from build123d import *

# Parameters (mm, degrees)
SKETCH1_R                = 7.5
SKETCH1_R_2              = 4
BOSS_EXTRUDE1_DEPTH      = 3
SKETCH2_R                = 8.5
SKETCH2_R_2              = 5.5
BOSS_EXTRUDE2_DEPTH      = 12
CUT_EXTRUDE1_DEPTH       = 17.985287751
CUT_EXTRUDE1_DEPTH_BACK  = 17.985287751
SKETCH4_R                = 1.5
BOSS_EXTRUDE4_DEPTH      = 6
BOSS_EXTRUDE4_DEPTH_BACK = 3
SKETCH5_R                = 8
SKETCH5_R_2              = 7


with BuildPart() as part:
    # Sketch1 → Boss-Extrude1 (new body)
    with BuildSketch(Plane.XY):
        Circle(SKETCH1_R)
        Circle(SKETCH1_R_2, mode=Mode.SUBTRACT)
    extrude(amount=BOSS_EXTRUDE1_DEPTH)

    # Sketch2 → Boss-Extrude2 (add)
    with BuildSketch(Plane.XY):
        Circle(SKETCH2_R)
        Circle(SKETCH2_R_2, mode=Mode.SUBTRACT)
    extrude(amount=-BOSS_EXTRUDE2_DEPTH)

    # Sketch4 → Cut-Extrude1 (cut, two sides: drawn at the far end of the back side and taken through both)
    with BuildSketch(Plane(origin=(0, 0, 0), x_dir=(0, 0, -1), z_dir=(1, 0, 0)).offset(-CUT_EXTRUDE1_DEPTH_BACK)):
        with Locations((7.5, 0)):
            Circle(SKETCH4_R)
    extrude(amount=CUT_EXTRUDE1_DEPTH + CUT_EXTRUDE1_DEPTH_BACK, mode=Mode.SUBTRACT)

    # Sketch5 → Boss-Extrude4 (add, two sides: drawn at the far end of the back side and taken through both)
    with BuildSketch(Plane.XY.offset(3).offset(-BOSS_EXTRUDE4_DEPTH_BACK)):
        Circle(SKETCH5_R)
        Circle(SKETCH5_R_2, mode=Mode.SUBTRACT)
    extrude(amount=BOSS_EXTRUDE4_DEPTH + BOSS_EXTRUDE4_DEPTH_BACK)


solid = part.part
Model file for the job. Use its own axes, mm. A direction names the side the tool comes from. Give positions to 0.01 mm unless a question says otherwise; leave off trailing zeros. Loops run counter-clockwise (first coordinate to the right, second up) from the corner with the lowest first, then second, coordinate; pieces in that order, holes last.
1) Saw through at B-B (x = 0). Write the cut outline in (y, z), plus the area to 3 significant figures.
2) Pull direction X, two halves, no side cores. Call faces 1 (the cylindrical face through (-1.73, -7.81, 4.44)), 2 (the cylindrical face through (-0.867, -3.905, 1.479)), 3 (the cylindrical face through (-6.918, -0.575, -8.886)): +X half, -X half, draft (parallel to the pull), parting line (faces both ways), or undercut.
3) Wall check: line 1 (Z direction, x = 7.4, y = 0); line 2 (X direction, y = 0, z = -4). Give the ranges that are in metal, low to high.
4) Saw through at D-D (z = -2.5). Write the cut outline in (x, y), plus the area to 3 significant figures.
5) Saw through at A-A (y = 0). Write the cut outline in (x, z).
6) Flat gauge pins, fed straight in: pin 1 Ø2 at (x, z) = (5, -5.5) entering from +Y; pin 2 Ø6.5 at (x, y) = (0, 0) entering from -Z; pin 3 Ø1 at (x, z) = (4, -2) entering from -Y; pin 4 Ø3.5 at (x, y) = (1, -2.5) entering from -Z. Where does each tip first touch, or does it go through?
7) Tool access for faces 4 (the flat face through (4, -6, 9)), 5 (the flat face through (-4, -2, 0)), 6 (the flat face through (3, -3, 3)): list every direction of +Z, -Z, +X, -X, +Y, -Y with a clear straight run to the whole face (end or side of a thin tool).
8) Saw through at C-C (z = -6.75). Write the cut outline in (x, y).
Answer block:
1. outline: (-8.5, -12) - (-5.5, -12) - (-5.5, 0) - (-4, 0) - (-4, 3) - (-7, 3) - (-7, 9) - (-8, 9) - (-8, 0) - (-8.5, 0) - close; (4, 0) - (5.5, 0) - (5.5, -12) - (8.5, -12) - (8.5, 0) - (8, 0) - (8, 9) - (7, 9) - (7, 3) - (4, 3) - close
1. area: 108 mm2
2. face 1: parting line
2. face 2: undercut
2. face 3: draft
3. line 1: z = -12 to -9, -6 to 9
3. line 2: x = -8.5 to -5.5, 5.5 to 8.5
4. outline: circle Ø17 at (0, 0); hole circle Ø11 at (0, 0)
4. area: 132 mm2
5. outline: (-8.5, -12) - (-5.5, -12) - (-5.5, -9) - (-8.5, -9) - close; (-8.5, -6) - (-5.5, -6) - (-5.5, 0) - (-4, 0) - (-4, 3) - (-7, 3) - (-7, 9) - (-8, 9) - (-8, 0) - (-8.5, 0) - close; (4, 0) - (5.5, 0) - (5.5, -6) - (8.5, -6) - (8.5, 0) - (8, 0) - (8, 9) - (7, 9) - (7, 3) - (4, 3) - close; (5.5, -12) - (8.5, -12) - (8.5, -9) - (5.5, -9) - close
6. pin 1: stops at y = 7.5
6. pin 2: passes through
6. pin 3: stops at y = -7.75
6. pin 4: stops at z = 0
7. face 4: +Z, +X, -X, +Y, -Y
7. face 5: -Z
7. face 6: +Z
8. outline: (-8.4, -1.3) arc R8.5 ccw to (8.4, -1.3) - (5.34, -1.3) arc R5.5 cw to (-5.34, -1.3) - close; (-8.4, 1.3) - (-5.34, 1.3) arc R5.5 cw to (5.34, 1.3) - (8.4, 1.3) arc R8.5 ccw to start
